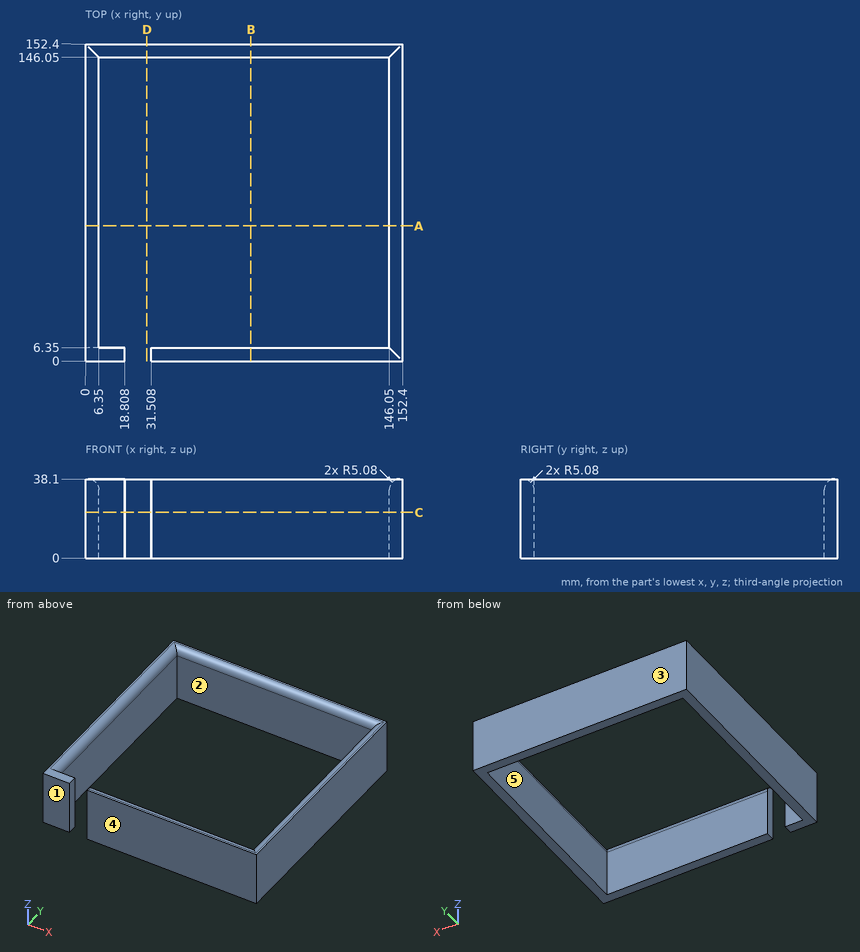
Here's the drawing with two shaded views (mm, measured from the low corner). I have some questions. A direction names the side the tool comes from. Coordinates: 2 decimals unless noted, no trailing zeros. Order: outer loops, then holes, each group sorted by start corner. A loop starts at its lowest first (then second) coordinate and runs counter-clockwise, first axis right, second up. Notation, with made-up numbers: M 51,-24.5 L 99,-24.5 A18 cw 99,9.5 Z; hole C 41.5,-15 d4. An arc over 180 degrees is marked long. Write item = value, one per line.
(1) Suppose I cut it at C-C on z = 22. Please give me the cut outline in (x, y).
Results are:
outline = M 0,0 L 18.81,0 L 18.81,6.35 L 6.35,6.35 L 6.35,146.05 L 146.05,146.05 L 146.05,6.35 L 31.51,6.35 L 31.51,0 L 152.4,0 L 152.4,152.4 L 0,152.4 Z
(2) Suppose I cut it at A-A on y = 65. Please give me the cut outline in (x, z), plus the area to 3 significant figures.
Results are:
outline = M 0,0 L 6.35,0 L 6.35,33.02 A5.08 ccw 1.27,38.1 L 0,38.1 Z; M 146.05,0 L 152.4,0 L 152.4,38.1 L 151.13,38.1 A5.08 ccw 146.05,33.02 Z
area = 473 mm2
(3) I need wall thicknesses on line 1 along Y through (x, z) = (95, 4); line 2 along X through (y, z) = (6, 4.5). Which ranges of each line are inside material? Lowest first, please. Write a range as [from, to].
Results are:
line_1 = [0, 6.35], [146.05, 152.4]
line_2 = [0, 18.81], [31.51, 152.4]
(4) Suppose I cut it at D-D on x = 29.5. Please give me the cut outline in (y, z), plus the area to 3 significant figures.
Results are:
outline = M 146.05,0 L 152.4,0 L 152.4,38.1 L 151.13,38.1 A5.08 ccw 146.05,33.02 Z
area = 236 mm2
(5) For the marked faces 4 and 5, which set-ups out of +Z, -Z, +X, -X, +Y, -Y let a thin tool reach every point of the face, with its end or its side?
Results are:
face_4 = +Z, -Z, +X, -X, -Y
face_5 = +Z, -Z
(6) If we mould it in two halves opening along Y, with no side actions, what happens to the marked faces 1, 2 and 3? For each: pulls with the +Y half, pulls with the -Y half, needs draft (parallel to the pull), parting line crosses it, or undercut.
Results are:
face_1 = pulls with the -Y half
face_2 = undercut
face_3 = pulls with the +Y half
